Check sheet for the drawn part. Datum: minimum x, y, z corner. Units: mm. Round coordinates to 2 decimals unless told otherwise and drop trailing zeros. Write each loop counter-clockwise with the first axis right and the second up, starting at its lowest first coordinate (ties: lowest second). Pieces come first, ordered by that corner, then holes. Notation, with made-up numbers: M 63.25,48 L 118.25,48 A18 cw 118.25,75 Z; hole C -25.5,61 d5. An arc over 180 degrees is marked long. Put each result on its own line as item: value.
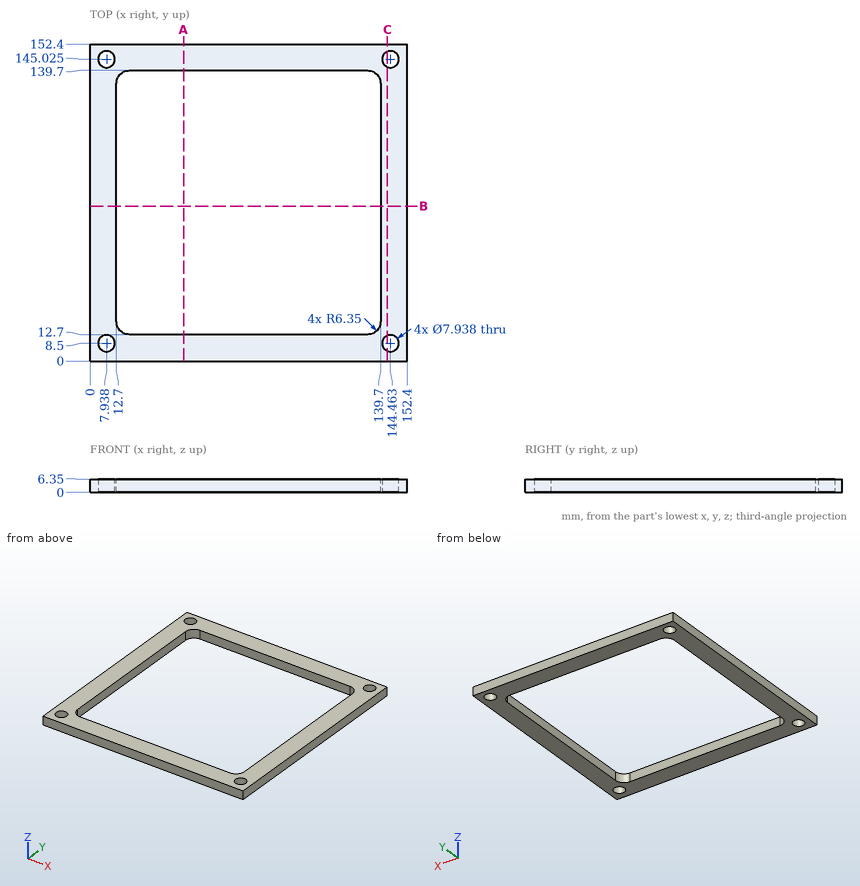
1. Depth check by flat-ended pin: pin 1 Ø7 at (x, y) = (144.46, 8.5) entering from -Z. Enter the tip coordinate at first touch or a pass-through.
Computed values:
pin 1: passes through
2. Cross-section at A-A (x = 45). Enter the section's corners in (y, z), then the cut area to 3 significant figures.
Computed values:
outline: M 0,0 L 12.7,0 L 12.7,6.35 L 0,6.35 Z; M 139.7,0 L 152.4,0 L 152.4,6.35 L 139.7,6.35 Z
area: 161 mm2
3. Scan lines: probe 1 along X at (y, z) = (8.5, 1.75); probe 2 along X at (y, z) = (64, 2.75). Record each from-to range of solid material in increasing order.
Computed values:
probe 1: x = 0 to 3.97, 11.91 to 140.49, 148.43 to 152.4
probe 2: x = 0 to 12.7, 139.7 to 152.4
4. Cross-section at C-C (x = 143). Count the separate pieces of the cut face and the enclosed holes in it, then the cut area to 3 significant figures.
Computed values:
separate pieces: 3
enclosed holes: 0
area: 874 mm2
